For this review, take the finished solid that the model builds, in its own axes (mm). Face numbers are marked on the shaded views. A direction names the side the tool comes from. Give positions to 0.01 mm unless a question says otherwise; leave off trailing zeros. Order: outer loops, then holes, each group sorted by start corner. A loop starts at its lowest first (then second) coordinate and runs counter-clockwise, first axis right, second up.
from build123d import *

# Parameters (mm, degrees)
SKETCH1_R                        = 20
BOSS_EXTRUDE1_DEPTH              = 40
SKETCH1_3_R                      = 20
BOSS_EXTRUDE2_DEPTH              = 30
SKETCH2_W                        = 80
SKETCH2_H                        = 40
BOSS_EXTRUDE3_DEPTH              = 10
SKETCH3_W                        = 80
SKETCH3_H                        = 10
BOSS_EXTRUDE4_DEPTH              = 30
BOSS_EXTRUDE5_DEPTH              = 10
CUT_EXTRUDE1_DEPTH               = 121.415945788
F_20_0MM_DOWEL_HOLE1_D           = 20
F_20_0MM_DOWEL_HOLE1_CSINK_D     = 20.05
F_20_0MM_DOWEL_HOLE1_CSINK_ANGLE = 100


with BuildPart() as part:
    # Sketch1 → Boss-Extrude1 (new body)
    with BuildSketch(Plane.XY):
        with Locations((-40, 0)):
            Circle(SKETCH1_R)
    extrude(amount=BOSS_EXTRUDE1_DEPTH)



with BuildPart() as body_2:
    # Sketch1<3> → Boss-Extrude2 (new body)
    with BuildSketch(Plane.XY):
        with Locations((40, 0)):
            Circle(SKETCH1_3_R)
    extrude(amount=BOSS_EXTRUDE2_DEPTH)


with BuildPart() as part_1:
    add(part.part)

    add(body_2.part)  # Boss-Extrude3 merges body 2
    # Sketch2 → Boss-Extrude3 (add)
    with BuildSketch(Plane(origin=(0, 0, 0), x_dir=(-1, 0, 0), z_dir=(0, 0, -1))):
        Rectangle(SKETCH2_W, SKETCH2_H)
    extrude(amount=-BOSS_EXTRUDE3_DEPTH)

    # Sketch3 → Boss-Extrude4 (add)
    with BuildSketch(Plane.XY.offset(30)):
        with Locations((0, -15)):
            Rectangle(SKETCH3_W, SKETCH3_H)
    extrude(amount=-BOSS_EXTRUDE4_DEPTH)

    # Sketch4 → Boss-Extrude5 (add)
    with BuildSketch(Plane(origin=(0, 0, 0), x_dir=(-1, 0, 0), z_dir=(0, 0, -1))):
        with BuildLine():
            Line((-30, -20), (30, -20))
            Line((30, -20), (30, -90))
            ThreePointArc((30, -90), (27.071067812, -97.071067812), (20, -100))
            Line((20, -100), (-20, -100))
            ThreePointArc((-20, -100), (-27.071067812, -97.071067812), (-30, -90))
            Line((-30, -90), (-30, -20))
        make_face()
    extrude(amount=-BOSS_EXTRUDE5_DEPTH)

    # Sketch5 → Cut-Extrude1 (cut, through all)
    with BuildSketch(Plane.XY.offset(10)):
        with BuildLine():
            Line((-5, -60), (10, -60))
            ThreePointArc((10, -60), (20, -70), (10, -80))
            Line((10, -80), (-5, -80))
            ThreePointArc((-5, -80), (-15, -70), (-5, -60))
        make_face()
    extrude(amount=-CUT_EXTRUDE1_DEPTH, mode=Mode.SUBTRACT)

    # Ø20.0mm Dowel Hole1 (through all)
    with Locations(Plane.XY.offset(40)):
        with Locations((-40, 0), (40, 0)):
            CounterSinkHole(F_20_0MM_DOWEL_HOLE1_D / 2, F_20_0MM_DOWEL_HOLE1_CSINK_D / 2, counter_sink_angle=F_20_0MM_DOWEL_HOLE1_CSINK_ANGLE)


solid = part_1.part
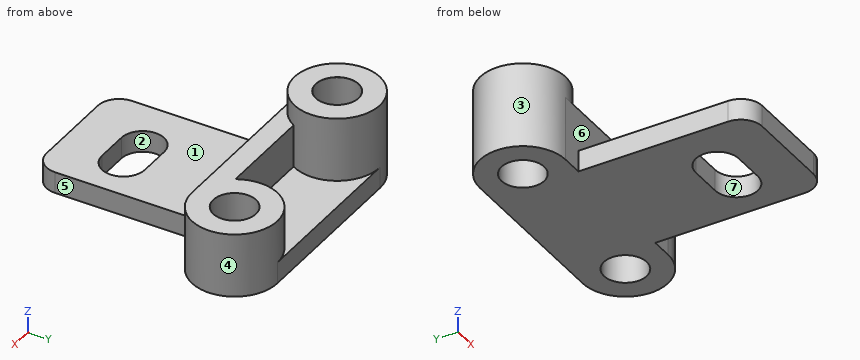
1) To check wall thickness, follow line 1 (Y direction, x = -40, z = 23); line 2 (Z direction, x = 22, y = -35); line 3 (Y direction, x = -4, z = 21.5). State the ranges of each line that lie inside material, in increasing order.
Answer sheet:
line 1: y = -20 to -10, 10 to 20
line 2: z = 0 to 10
line 3: y = -20 to -10
2) Draft analysis for pull direction X (two halves, no side actions). For the marked faces 4, 5, 6 and 7, state which applies: +X half, -X half, draft (parallel to the pull), parting line (faces both ways), or undercut.
Answer sheet:
face 4: undercut
face 5: +X half
face 6: draft
face 7: undercut
3) Clearance check with flat-ended pins moving along their axes: pin 1 (2 mm diameter, centred on y = -28, z = 6, fed in from -X); pin 2 (1 mm diameter, centred on x = 38, z = 15, fed in from -Y); pin 3 (11 mm diameter, centred on y = -57, z = 3, fed in from +X); pin 4 (4 mm diameter, centred on x = -33, y = -79.5, fed in from -Z). State where each tip first meets the part, or that it passes through.
Answer sheet:
pin 1: stops at x = -30
pin 2: stops at y = -20
pin 3: stops at x = 30
pin 4: passes through
4) We need section A-A on y = 0. Give the boundary of the cut face in (x, z) (3 decimals).
Answer sheet:
outline: (-60, 0) - (-50, 0) - (-50, 39.979) - (-50.025, 40) - (-60, 40) - close; (-30, 0) - (30, 0) - (30, 30) - (20, 30) - (20, 10) - (-20, 10) - (-20, 40) - (-29.975, 40) - (-30, 39.979) - close; (50, 0) - (60, 0) - (60, 30) - (50, 30) - close
5) We need section D-D on x = 28.5. Give the boundary of the cut face in (y, z).
Answer sheet:
outline: (-95.27, 0) - (20, 0) - (20, 10) - (16.36, 10) - (16.36, 30) - (-20, 30) - (-20, 10) - (-95.27, 10) - close
6) We need section B-B on y = -70. Give the boundary of the cut face in (x, z).
Answer sheet:
outline: (-30, 0) - (-15, 0) - (-15, 10) - (-30, 10) - close; (20, 0) - (30, 0) - (30, 10) - (20, 10) - close
7) We need section C-C on z = 13. Give the boundary of the cut face in (x, y).
Answer sheet:
outline: (-40, -20) - (40, -20) arc R20 ccw (long way) to (22.68, -10) - (-22.68, -10) arc R20 ccw (long way) to start; hole circle Ø20 at (-40, 0); hole circle Ø20 at (40, 0)
8) Tool access review of the marked faces 1, 2 and 3: name each direction out of +Z, -Z, +X, -X, +Y, -Y from which nothing blocks a thin tool from reaching the whole face with its end or side.
Answer sheet:
face 1: +Z, +X, -X, -Y
face 2: +Z, -Z
face 3: +Z
